```python
from build123d import *

# Parameters (mm, degrees)
CUT_EXTRUDE1_REACH  = 28.096
SKETCH5_R           = 14
SKETCH5_R_2         = 11.878679656
BOSS_EXTRUDE2_DEPTH = 5
BOSS_EXTRUDE3_START = -1
SKETCH3_W           = 3.7
SKETCH3_H           = 1.8
BOSS_EXTRUDE3_DEPTH = 7


with BuildPart() as part:
    # Sketch1 → Revolve1 (revolve)
    with BuildSketch(Plane.XY, mode=Mode.PRIVATE) as revolve1_sk:
        Polygon((14, 0), (14, 9), (6, 17), (2.6, 17), (2.6, 18), (1.5, 18), (1.5, 9), (2.5, 9), (2.5, 10), (4.5, 12), (8.878679656, 12), (13.5, 7.378679656), (13.5, 0), align=None)
    revolve(revolve1_sk.sketch.rotate(Axis((0, 0, 0), (0, 1, 0)), 90), axis=Axis((0, 0, 0), (0, 1, 0)))

    # Cut-Extrude1: up to this face of the body (flat: up to its plane)
    cut_extrude1_end = Plane(part.part.faces().sort_by_distance((0, 9, 1.570710678))[0])
    # Sketch2 → Cut-Extrude1 (cut, up to the picked face)
    with BuildSketch(Plane(origin=(0, 17, 0), x_dir=(1, 0, 0), z_dir=(0, 1, 0)), mode=Mode.PRIVATE) as cut_extrude1_sk1:
        with BuildLine():
            Line((3.5, 13.555441712), (1.969238681, 7.626828615))
            ThreePointArc((1.969238681, 7.626828615), (3.181980515, 3.181980515), (7.626828615, 1.969238681))
            Line((7.626828615, 1.969238681), (13.555441712, 3.5))
            ThreePointArc((13.555441712, 3.5), (9.899494937, 9.899494937), (3.5, 13.555441712))
        make_face()
    cut_extrude1_tool1 = split(extrude(cut_extrude1_sk1.sketch, amount=-CUT_EXTRUDE1_REACH, mode=Mode.PRIVATE), bisect_by=cut_extrude1_end, keep=Keep.BOTH, mode=Mode.PRIVATE)
    # Sketch2 → Cut-Extrude1 (cut, up to the picked face)
    with BuildSketch(Plane(origin=(0, 17, 0), x_dir=(1, 0, 0), z_dir=(0, 1, 0)), mode=Mode.PRIVATE) as cut_extrude1_sk2:
        with BuildLine():
            Line((13.555441712, -3.5), (7.626828615, -1.969238681))
            ThreePointArc((7.626828615, -1.969238681), (3.181980515, -3.181980515), (1.969238681, -7.626828615))
            Line((1.969238681, -7.626828615), (3.5, -13.555441712))
            ThreePointArc((3.5, -13.555441712), (9.899494937, -9.899494937), (13.555441712, -3.5))
        make_face()
    cut_extrude1_tool2 = split(extrude(cut_extrude1_sk2.sketch, amount=-CUT_EXTRUDE1_REACH, mode=Mode.PRIVATE), bisect_by=cut_extrude1_end, keep=Keep.BOTH, mode=Mode.PRIVATE)
    # Sketch2 → Cut-Extrude1 (cut, up to the picked face)
    with BuildSketch(Plane(origin=(0, 17, 0), x_dir=(1, 0, 0), z_dir=(0, 1, 0)), mode=Mode.PRIVATE) as cut_extrude1_sk3:
        with BuildLine():
            Line((-3.5, -13.555441712), (-1.969238681, -7.626828615))
            ThreePointArc((-1.969238681, -7.626828615), (-3.181980515, -3.181980515), (-7.626828615, -1.969238681))
            Line((-7.626828615, -1.969238681), (-13.555441712, -3.5))
            ThreePointArc((-13.555441712, -3.5), (-9.899494937, -9.899494937), (-3.5, -13.555441712))
        make_face()
    cut_extrude1_tool3 = split(extrude(cut_extrude1_sk3.sketch, amount=-CUT_EXTRUDE1_REACH, mode=Mode.PRIVATE), bisect_by=cut_extrude1_end, keep=Keep.BOTH, mode=Mode.PRIVATE)
    # Sketch2 → Cut-Extrude1 (cut, up to the picked face)
    with BuildSketch(Plane(origin=(0, 17, 0), x_dir=(1, 0, 0), z_dir=(0, 1, 0)), mode=Mode.PRIVATE) as cut_extrude1_sk4:
        with BuildLine():
            Line((-13.555441712, 3.5), (-7.626828615, 1.969238681))
            ThreePointArc((-7.626828615, 1.969238681), (-3.181980515, 3.181980515), (-1.969238681, 7.626828615))
            Line((-1.969238681, 7.626828615), (-3.5, 13.555441712))
            ThreePointArc((-3.5, 13.555441712), (-9.899494937, 9.899494937), (-13.555441712, 3.5))
        make_face()
    cut_extrude1_tool4 = split(extrude(cut_extrude1_sk4.sketch, amount=-CUT_EXTRUDE1_REACH, mode=Mode.PRIVATE), bisect_by=cut_extrude1_end, keep=Keep.BOTH, mode=Mode.PRIVATE)
    add(cut_extrude1_tool1.solids().sort_by(Axis((6.913029, 17, -6.913029), (0, -1, 0)))[0], mode=Mode.SUBTRACT)
    add(cut_extrude1_tool2.solids().sort_by(Axis((6.913029, 17, 6.913029), (0, -1, 0)))[0], mode=Mode.SUBTRACT)
    add(cut_extrude1_tool3.solids().sort_by(Axis((-6.913029, 17, 6.913029), (0, -1, 0)))[0], mode=Mode.SUBTRACT)
    add(cut_extrude1_tool4.solids().sort_by(Axis((-6.913029, 17, -6.913029), (0, -1, 0)))[0], mode=Mode.SUBTRACT)

    # Sketch5 → Boss-Extrude2 (add)
    with BuildSketch(Plane(origin=(0, 9, 0), x_dir=(1, 0, 0), z_dir=(0, 1, 0))):
        with Locations(Location((0, 0, 0), (0, 0, 90))):
            Circle(SKETCH5_R)
        with Locations(Location((0, 0, 0), (0, 0, 284.477512186))):
            Circle(SKETCH5_R_2, mode=Mode.SUBTRACT)
    extrude(amount=-BOSS_EXTRUDE2_DEPTH)

    # Sketch3 → Boss-Extrude3 (add)
    with BuildSketch(Plane.XZ.offset(BOSS_EXTRUDE3_START)):
        with Locations((0, 12.6)):
            Rectangle(SKETCH3_W, SKETCH3_H)
        Polygon((3.409647342, 11.344020672), (6.743232153, 9.738650837), (7.524222884, 11.360394799), (4.190638072, 12.965764634), align=None)
        Polygon((7.993972211, 8.741218924), (10.300884478, 5.848442439), (11.708181147, 6.970724083), (9.40126888, 9.863500568), align=None)
        Polygon((10.994992845, 4.407111565), (11.8183203, 0.79987829), (13.573190542, 1.200415971), (12.749863087, 4.807649246), align=None)
        Polygon((11.8183203, -0.79987829), (10.994992845, -4.407111565), (12.749863087, -4.807649246), (13.573190542, -1.200415971), align=None)
        Polygon((10.300884478, -5.848442439), (7.993972211, -8.741218924), (9.40126888, -9.863500568), (11.708181147, -6.970724083), align=None)
        Polygon((6.743232153, -9.738650837), (3.409647342, -11.344020672), (4.190638072, -12.965764634), (7.524222884, -11.360394799), align=None)
        with Locations((0, -12.6)):
            Rectangle(SKETCH3_W, SKETCH3_H)
        Polygon((-3.409647342, -11.344020672), (-6.743232153, -9.738650837), (-7.524222884, -11.360394799), (-4.190638072, -12.965764634), align=None)
        Polygon((-7.993972211, -8.741218924), (-10.300884478, -5.848442439), (-11.708181147, -6.970724083), (-9.40126888, -9.863500568), align=None)
        Polygon((-10.994992845, -4.407111565), (-11.8183203, -0.79987829), (-13.573190542, -1.200415971), (-12.749863087, -4.807649246), align=None)
        Polygon((-11.8183203, 0.79987829), (-10.994992845, 4.407111565), (-12.749863087, 4.807649246), (-13.573190542, 1.200415971), align=None)
        Polygon((-10.300884478, 5.848442439), (-7.993972211, 8.741218924), (-9.40126888, 9.863500568), (-11.708181147, 6.970724083), align=None)
        Polygon((-6.743232153, 9.738650837), (-3.409647342, 11.344020672), (-4.190638072, 12.965764634), (-7.524222884, 11.360394799), align=None)
    extrude(amount=-BOSS_EXTRUDE3_DEPTH)


solid = part.part
```
Input: part model. Units: mm. Frame: model coordinates. A direction names the side the tool comes from. Round coordinates to 2 decimals unless told otherwise and drop trailing zeros. Loops run counter-clockwise (first coordinate to the right, second up) from the corner with the lowest first, then second, coordinate; pieces in that order, holes last. Notation, with made-up numbers: (-24, 66.25) -> (-4, 66.25) arc R31 cw to (-4, 90.25) -> close; hole circle Ø4 at (-22.75, 32). An arc over 180 degrees is marked (long way). Use one line per item in the form item = value. Start each with the question number.
Item 1: Set-up query: faces 1 (the face through (9.92, 11.62, -2.56)), 2 (the face through (2.57, 11.4, -9.95)), 3 (the face through (3.23, 14.535, 3.135)), 4 (the face through (8, 4, 10)), 5 (the face through (-10, 13, 0)). Return all of +Z, -Z, +X, -X, +Y, -Y with unobstructed straight access to the full face (end or side cutting, diameter ignored); none if empty.
Item 2: Contact query for flat-ended pins moving along their axis: pin 1 Ø1.1 at (x, z) = (11.5, 5.5) entering from -Y; pin 2 Ø1 at (x, z) = (1, 2) entering from -Y; pin 3 Ø1.3 at (x, z) = (5, -10.5) entering from +Y. Output: stop coordinate, or through.
Item 3: Section query D-D on y = 14.75. Return the cut outline in (x, z).
Item 4: Material intervals for L1, parallel to X at y = 1.7, z = 0; L2, parallel to Y at x = -9.75, z = -7.25; L3, parallel to Y at x = 10.75, z = -5.25, sorted ascending. Write a range as from..to.
Item 5: Section query C-C on y = 11. Return the cut outline in (x, z) (3 decimals).
Ans:
q1.face_1 = -Z, +Y
q1.face_2 = +X, +Y
q1.face_3 = +Y, -Y
q1.face_4 = -Y
q1.face_5 = -X, +Y
q2.pin_1 = 4
q2.pin_2 = 9
q2.pin_3 = 9
q3.outline = (-7.99, -2.06) -> (-7.63, -1.97) arc R4.64 cw to (-1.97, -7.63) -> (-2.06, -7.99) arc R8.25 ccw to (2.06, -7.99) -> (1.97, -7.63) arc R4.64 cw to (7.63, -1.97) -> (7.99, -2.06) arc R8.25 ccw to (7.99, 2.06) -> (7.63, 1.97) arc R4.64 cw to (1.97, 7.63) -> (2.06, 7.99) arc R8.25 ccw to (-2.06, 7.99) -> (-1.97, 7.63) arc R4.64 cw to (-7.63, 1.97) -> (-7.99, 2.06) arc R8.25 ccw to start; hole circle Ø3 at (0, 0)
q4.L1 = -14..-13.5, 13.5..14
q4.L2 = 1..9
q4.L3 = 4..9
q5.outline = (-11.619, -3) -> (-9.565, -2.47) arc R9.879 cw to (-9.565, 2.47) -> (-11.619, 3) arc R12 ccw to start; circle Ø7 at (0, 0); (-3, -11.619) arc R12 ccw to (3, -11.619) -> (2.47, -9.565) arc R9.879 cw to (-2.47, -9.565) -> close; (-3, 11.619) -> (-2.47, 9.565) arc R9.879 cw to (2.47, 9.565) -> (3, 11.619) arc R12 ccw to start; (9.565, -2.47) -> (11.619, -3) arc R12 ccw to (11.619, 3) -> (9.565, 2.47) arc R9.879 cw to start; hole circle Ø3 at (0, 0)
